Study the drawing (mm; zero at the part's minimum x, y, z) and answer. Give positions to 0.01 mm unless a question says otherwise; leave off trailing zeros. Write each loop counter-clockwise with the first axis right and the second up, starting at its lowest first coordinate (ties: lowest second). Pieces come first, ordered by that corner, then holes. Notation, with made-up numbers: (69.25, 1) - (99.25, 1) arc R11 ccw to (99.25, 5) - close; hole circle Ø10 at (-32, 63.5). An arc over 180 degrees is marked (long way). Return JSON: item names as keys, results as strings.
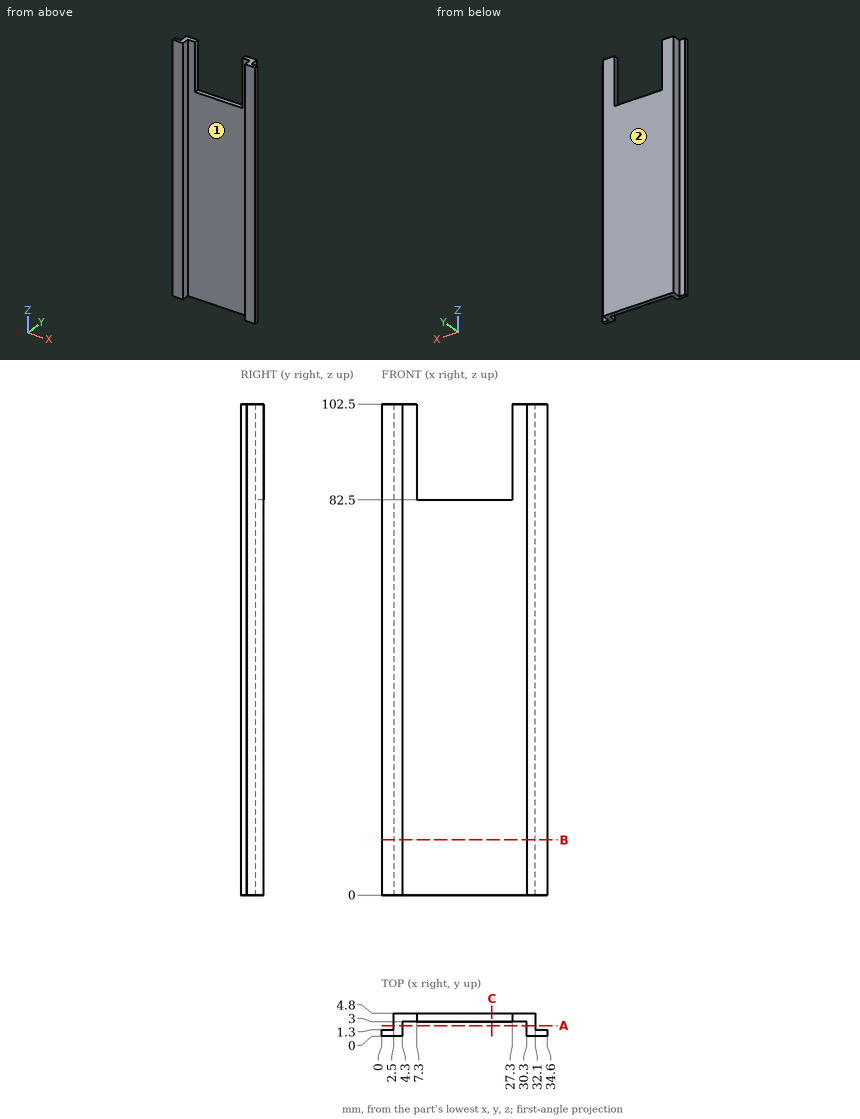
Item 1: Flat-ended cylindrical pins translate along their axes: P1, Ø8, axis at x = 16.5, z = 70.5, coming from the -Y side; P2, Ø1, axis at y = 3, z = 45.5, coming from the -X side; P3, Ø2, axis at y = 3.5, z = 92.5, coming from the +X side. Find the tip coordinate at first contact, or state that the pin passes through.
Answer below:
{"P1": "stops at y = 3", "P2": "stops at x = 2.5", "P3": "stops at x = 32.1"}
Item 2: A cutting plane is placed at C-C on x = 23. Determine the outline of the cut face in (y, z).
Answer below:
{"outline": "(3, 0) - (4.8, 0) - (4.8, 82.5) - (3, 82.5) - close"}
Item 3: A cutting plane is placed at B-B on z = 11.5. Determine the outline of the cut face in (x, y), then the cut area to 3 significant figures.
Answer below:
{"outline": "(0, 0) - (4.3, 0) - (4.3, 3) - (30.3, 3) - (30.3, 0) - (34.6, 0) - (34.6, 1.3) - (32.1, 1.3) - (32.1, 4.8) - (2.5, 4.8) - (2.5, 1.3) - (0, 1.3) - close", "area": "70.6 mm²"}
Item 4: A cutting plane is placed at A-A on y = 2.15. Determine the outline of the cut face in (x, z), then the cut area to 3 significant figures.
Answer below:
{"outline": "(2.5, 0) - (4.3, 0) - (4.3, 102.5) - (2.5, 102.5) - close; (30.3, 0) - (32.1, 0) - (32.1, 102.5) - (30.3, 102.5) - close", "area": "369 mm²"}
Item 5: The mould has two halves that part along X. Classify the marked faces 1 and 2: +X half, -X half, draft (parallel to the pull), parting line (faces both ways), or undercut.
Answer below:
{"face 1": "undercut", "face 2": "draft"}
Item 6: Consider L1, parallel to X at y = 1.5, z = 86; L2, parallel to X at y = 0.7, z = 46; L3, parallel to Y at x = 19.5, z = 71. Determine where each line is inside the solid, lowest interval first.
Answer below:
{"L1": "x = 2.5 to 4.3, 30.3 to 32.1", "L2": "x = 0 to 4.3, 30.3 to 34.6", "L3": "y = 3 to 4.8"}
